Could you check a few things on this model? Use its own coordinates, in mm. A direction names the side the tool comes from. Give positions to 0.01 mm unless a question says otherwise; leave off trailing zeros. Write each loop counter-clockwise with the first axis right and the second up, starting at its lowest first coordinate (ties: lowest second). Pieces come first, ordered by that corner, then holes. Notation, with made-up numbers: M 47.25,86.25 L 105.25,86.25 A16 cw 105.25,111.25 Z; hole C 10.25,25 d6. An arc over 180 degrees is marked long. Use one line per item in the form item = value.
from build123d import *

# Parameters (mm, degrees)
SKETCH_W             = 60
SKETCH_H             = 60
PAD_DEPTH            = 4
SKETCH001_R          = 3.5
SKETCH001_R_2        = 1.25
PAD001_DEPTH         = 8
SKETCH009_W          = 5
SKETCH009_H          = 25
POCKET008_DEPTH      = 4
PAD006_DEPTH         = 4
SKETCH015_W          = 22
SKETCH015_H          = 4
PAD007_DEPTH         = 2
SKETCH003_R          = 2.25
PAD008_DEPTH         = 8
SKETCH014_R          = 3.5
SKETCH014_R_2        = 1.25
PAD009_DEPTH         = 15
POCKET_DEPTH         = 4
BODY_PLACEMENT_ANGLE = 195


with BuildPart() as part:
    # Sketch → Pad (new body)
    with BuildSketch(Plane.XY):
        Rectangle(SKETCH_W, SKETCH_H)
    extrude(amount=PAD_DEPTH)

    # Sketch001 (on Face6 of Pad) → Pad001 (join)
    with BuildSketch(Plane.XY.offset(4)):
        with Locations((-17, 17)):
            Circle(SKETCH001_R)
        with Locations((-17, 17)):
            Circle(SKETCH001_R_2, mode=Mode.SUBTRACT)
        with Locations((-17, -17)):
            Circle(SKETCH001_R)
        with Locations((-17, -17)):
            Circle(SKETCH001_R_2, mode=Mode.SUBTRACT)
        with Locations((17, -17)):
            Circle(SKETCH001_R)
        with Locations((17, -17)):
            Circle(SKETCH001_R_2, mode=Mode.SUBTRACT)
        with Locations((17, 17)):
            Circle(SKETCH001_R)
        with Locations((17, 17)):
            Circle(SKETCH001_R_2, mode=Mode.SUBTRACT)
    extrude(amount=PAD001_DEPTH)

    # Sketch009 → Pocket008 (cut)
    with BuildSketch(Plane(origin=(0, 0, 0), x_dir=(1, 0, 0), z_dir=(0, 0, -1))):
        Rectangle(SKETCH009_W, SKETCH009_H)
        with Locations((10, 0)):
            Rectangle(SKETCH009_W, SKETCH009_H)
        with Locations((20, 0)):
            Rectangle(SKETCH009_W, SKETCH009_H)
        with Locations((-10, 0)):
            Rectangle(SKETCH009_W, SKETCH009_H)
        with Locations((-20, 0)):
            Rectangle(SKETCH009_W, SKETCH009_H)
    extrude(amount=-POCKET008_DEPTH, mode=Mode.SUBTRACT)

    # Sketch012 (on Face5 of Pocket008) → Pad006 (join)
    with BuildSketch(Plane.XY.offset(4)):
        Polygon((-30, -12), (-35, -12), (-35, -30), (-33, -28), (-33, -16), (-30, -16), align=None)
    pad006 = extrude(amount=-PAD006_DEPTH)

    # Mirrored005: Pad006 across Sketch012 V_Axis
    add(pad006.mirror(Plane(origin=(0, 0, 4), x_dir=(0, 0, 1), z_dir=(1, 0, 0))))

    # Sketch015 (on Face4 of Pad) → Pad007 (join)
    with BuildSketch(Plane(origin=(-30, 0, 0), x_dir=(0, -1, 0), z_dir=(-1, 0, 0))):
        with Locations((0, 2)):
            Rectangle(SKETCH015_W, SKETCH015_H)
    pad007 = extrude(amount=PAD007_DEPTH)

    # Sketch003 (on Face42 of Pad007) → Pad008 (join)
    with BuildSketch(Plane(origin=(-32, 0, 0), x_dir=(0, -1, 0), z_dir=(-1, 0, 0))):
        with BuildLine():
            ThreePointArc((11, 19), (0, 25.938622), (-11, 19))
            Line((-11, 19), (-11, 0))
            Line((11, 0), (-11, 0))
            Line((11, 19), (11, 0))
        make_face()
        with Locations((0, 13.75)):
            Circle(SKETCH003_R, mode=Mode.SUBTRACT)
    pad008 = extrude(amount=PAD008_DEPTH)

    # Sketch014 → Pad009 (join)
    with BuildSketch(Plane.XY.offset(4)):
        with Locations((-23.5, 23.5)):
            Circle(SKETCH014_R)
        with Locations((-23.5, 23.5)):
            Circle(SKETCH014_R_2, mode=Mode.SUBTRACT)
        with Locations((23.5, 23.5)):
            Circle(SKETCH014_R)
        with Locations((23.5, 23.5)):
            Circle(SKETCH014_R_2, mode=Mode.SUBTRACT)
        with Locations((23.5, -23.5)):
            Circle(SKETCH014_R)
        with Locations((23.5, -23.5)):
            Circle(SKETCH014_R_2, mode=Mode.SUBTRACT)
        with Locations((-23.5, -23.5)):
            Circle(SKETCH014_R)
        with Locations((-23.5, -23.5)):
            Circle(SKETCH014_R_2, mode=Mode.SUBTRACT)
    extrude(amount=PAD009_DEPTH)

    # Sketch016 (on Face58 of Pad009) → Pocket (cut)
    with BuildSketch(Plane.YZ.offset(-32)):
        Polygon((-3.637307, 15.85), (-3.637307, 11.65), (0, 9.55), (3.637307, 11.65), (3.637307, 15.85), (0, 17.95), align=None)
    pocket = extrude(amount=-POCKET_DEPTH, mode=Mode.SUBTRACT)

    # Mirrored: Pad007, Pad008 across YZ
    add(pad007.mirror(Plane.YZ))
    add(pad008.mirror(Plane.YZ))

    # Mirrored006: Pocket across YZ
    add(pocket.mirror(Plane.YZ), mode=Mode.SUBTRACT)


with BuildPart() as part_1:
    # Body placement: moved
    add(part.part.moved(Location((0, 44.339027, 22.284409))).rotate(Axis((0, 44.339027, 22.284409), (1, 0, 0)), BODY_PLACEMENT_ANGLE))


solid = part_1.part
1) For faces 1 (the flat face through (-31.521, 60.319, 24.467)), 2 (the flat face through (35, 65, 26)), 3 (the flat face through (-36.041, 57.457, 15.827)), 4 (the flat face through (-33.972, 51.419, 9.916)), 5 (the flat face through (-32, 51, 6)), which set-ups out of +Z, -Z, +X, -X, +Y, -Y let a thin tool reach every point of the face, with its end or its side?
Checked values:
face_1 = +Z, +Y
face_2 = +Z, +X, +Y
face_3 = -X
face_4 = none
face_5 = -Z, +Y
2) For pin 1 Ø5 at (x, y) = (12.5, 56) entering from +Z; pin 2 Ø3 at (x, z) = (28, 5) entering from -Y; pin 3 Ø7.5 at (y, z) = (68, 25) entering from -X, each with a flat end and sliding along its axis, tell me the tip position at first contact or that it passes through.
Checked values:
pin_1 = 26.08
pin_2 = 22.74
pin_3 = -35
3) If I drill on L1, parallel to X at y = 44, z = 18.5; L2, parallel to X at y = 70.5, z = 26; L3, parallel to X at y = 70.5, z = 17.5, over which ranges is the centre line in solid material (lowest first)?
Checked values:
L1 = -40 to -22.5, -17.5 to -12.5, -7.5 to -2.5, 2.5 to 7.5, 12.5 to 17.5, 22.5 to 40
L2 = -35 to -33, -30 to 30, 33 to 35
L3 = -26.96 to -24.63, -22.37 to -20.04, 20.04 to 22.37, 24.63 to 26.96
4) I want a section at C-C, the plane y = 39.5. Please give me the cut outline in (x, z), plus the area to 3 significant figures.
Checked values:
outline = M -40,0.17 L -32,0.17 L -32,16.85 L -22.5,16.85 L -22.5,20.99 L -40,20.99 Z; M -17.5,16.85 L -12.5,16.85 L -12.5,20.99 L -17.5,20.99 Z; M -7.5,16.85 L -2.5,16.85 L -2.5,20.99 L -7.5,20.99 Z; M 2.5,16.85 L 7.5,16.85 L 7.5,20.99 L 2.5,20.99 Z; M 12.5,16.85 L 17.5,16.85 L 17.5,20.99 L 12.5,20.99 Z; M 22.5,16.85 L 32,16.85 L 32,0.17 L 40,0.17 L 40,20.99 L 22.5,20.99 Z
area = 495 mm2
5) Thinking about a two-plate mould opening in Z: for faces 6 (the flat face through (16.982, 61.778, 22.816)), 7 (the cylindrical face through (-35.94, 51.24, -2.72)), 8 (the flat face through (-10.035, 32.775, 17.144)), which applies, released by +Z, released by -Z, zero draft, split by the parting line, or undercut?
Checked values:
face_6 = undercut
face_7 = released by -Z
face_8 = released by +Z
6) I want a section at A-A, the plane x = -34. Please give me the cut outline in (y, z).
Checked values:
outline = M 33.71,19.44 L 38.63,1.08 A12.19 ccw 59.88,6.78 L 54.96,25.13 Z; M 55.93,25.39 L 56.97,21.53 L 73.39,25.93 L 72.35,29.79 Z; hole M 43.84,10.09 L 44.93,6.03 L 48.98,4.95 L 51.95,7.92 L 50.87,11.97 L 46.81,13.06 Z
7) I want a section at B-B, the plane x = 11.5. Please give me the cut outline in (y, z).
Checked values:
outline = M 15.36,14.52 L 16.4,10.66 L 33.3,15.19 L 32.26,19.05 Z; M 56.41,25.52 L 57.45,21.66 L 74.35,26.19 L 73.32,30.05 Z
8) I want a section at D-D, the plane z = 17. Count the separate pieces of the cut face and the enclosed holes in it, plus the area to 3 significant figures.
Checked values:
separate_pieces = 5
enclosed_holes = 4
area = 1,270 mm2
